from build123d import *

# Parameters (mm, degrees)
F0_W     = 152.4
F0_H     = 12.7
F0_W_2   = 12.7
F0_W_3   = 368.3
F1_DEPTH = 11.43
F2_DEPTH = 11.684


with BuildPart() as f1:
    # F0 (on Top) → F1 (new body)
    with BuildSketch(Plane.XY):
        with Locations((-273.05, 0)):
            Rectangle(F0_W, F0_H)
        with Locations((-190.5, 0)):
            Rectangle(F0_W_2, F0_H)
        with Locations((-177.8, 0)):
            Rectangle(F0_W_2, F0_H)
        with Locations((-165.1, 0)):
            Rectangle(F0_W_2, F0_H)
        with Locations((-152.4, 0)):
            Rectangle(F0_W_2, F0_H)
        with Locations((-139.7, 0)):
            Rectangle(F0_W_2, F0_H)
        with Locations((-127, 0)):
            Rectangle(F0_W_2, F0_H)
        with Locations((-114.3, 0)):
            Rectangle(F0_W_2, F0_H)
        with Locations((-101.6, 0)):
            Rectangle(F0_W_2, F0_H)
        with Locations((-88.9, 0)):
            Rectangle(F0_W_2, F0_H)
        with Locations((-76.2, 0)):
            Rectangle(F0_W_2, F0_H)
        with Locations((-63.5, 0)):
            Rectangle(F0_W_2, F0_H)
        with Locations((-50.8, 0)):
            Rectangle(F0_W_2, F0_H)
        with Locations((-38.1, 0)):
            Rectangle(F0_W_2, F0_H)
        with Locations((-25.4, 0)):
            Rectangle(F0_W_2, F0_H)
        with Locations((165.1, 0)):
            Rectangle(F0_W_3, F0_H)
    extrude(amount=F1_DEPTH)

    # F0 (on Top) → F2 (join)
    with BuildSketch(Plane.XY):
        with Locations((-190.5, 0)):
            Rectangle(F0_W_2, F0_H)
        with Locations((-165.1, 0)):
            Rectangle(F0_W_2, F0_H)
        with Locations((-139.7, 0)):
            Rectangle(F0_W_2, F0_H)
        with Locations((-114.3, 0)):
            Rectangle(F0_W_2, F0_H)
        with Locations((-88.9, 0)):
            Rectangle(F0_W_2, F0_H)
    extrude(amount=F2_DEPTH)


solid = f1.part
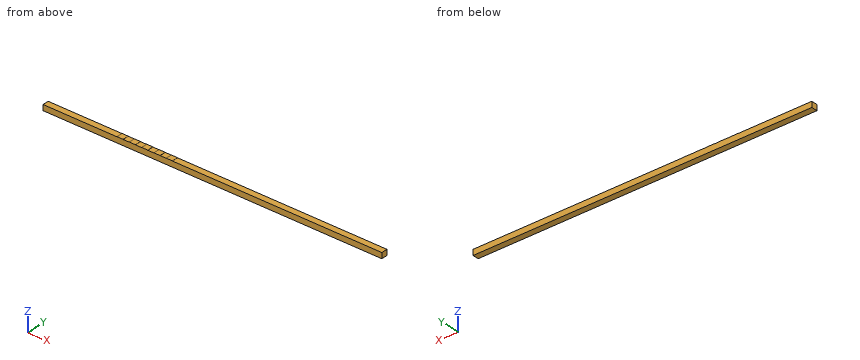
Here's how the part is built. I have some questions about the finished solid (model axes, mm). Round coordinates to 2 decimals unless told otherwise and drop trailing zeros. Loops run counter-clockwise (first coordinate to the right, second up) from the corner with the lowest first, then second, coordinate; pieces in that order, holes last. Notation, with made-up numbers: M -24,-24.5 L 28,-24.5 A28 ccw 28,9.5 Z; hole C -37,82 d10. An arc over 180 degrees is marked long. Write each question's results on one line, items separated by ' | '. Start each with the question number.
(1) I want a section at A-A (y = -0.5). Please give me the cut outline in (x, z), then the cut area to 3 significant figures.
(2) I want a section at B-B (x = 97.5). Please give me the cut outline in (y, z).
(3) If I drill on probe 1 along Z at (x, y) = (69, 4.5), over which ranges is the centre line in solid material (lowest first)? Write a range as from..to.
(4) Will this pin go through, and if not, where does the flat tip stop? P1, Ø4, axis at x = -249, y = 0, coming from the +Z side.
Solved:
1) outline: M -349.25,0 L 349.25,0 L 349.25,11.43 L -82.55,11.43 L -82.55,11.68 L -95.25,11.68 L -95.25,11.43 L -107.95,11.43 L -107.95,11.68 L -120.65,11.68 L -120.65,11.43 L -133.35,11.43 L -133.35,11.68 L -146.05,11.68 L -146.05,11.43 L -158.75,11.43 L -158.75,11.68 L -171.45,11.68 L -171.45,11.43 L -184.15,11.43 L -184.15,11.68 L -196.85,11.68 L -196.85,11.43 L -349.25,11.43 Z | area: 8,000 mm²
2) outline: M -6.35,0 L 6.35,0 L 6.35,11.43 L -6.35,11.43 Z
3) probe 1: z = 0..11.43
4) P1: stops at z = 11.43
